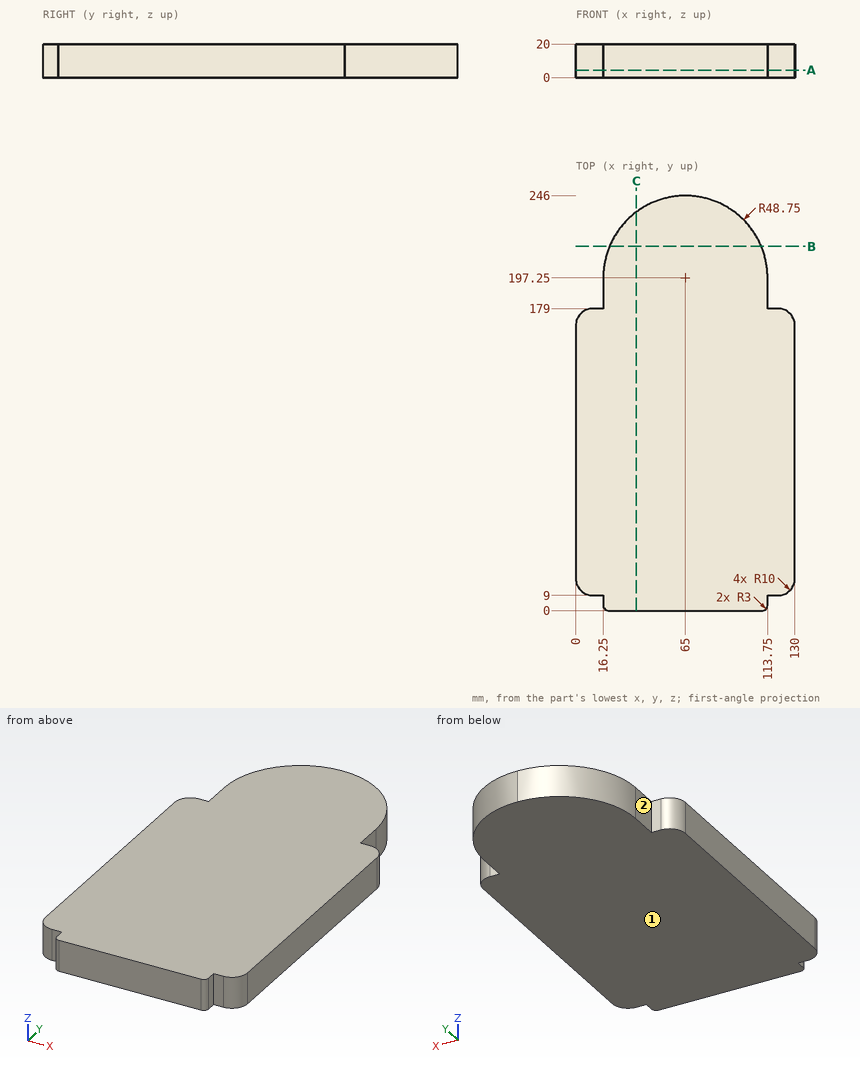
Geometry check sheet. Reference: drawing and pictorial views, mm from the part's lowest x, y, z. A direction names the side the tool comes from. Round coordinates to 2 decimals unless told otherwise and drop trailing zeros. Loops run counter-clockwise (first coordinate to the right, second up) from the corner with the lowest first, then second, coordinate; pieces in that order, holes last. Notation, with made-up numbers: (17.25, 16) -> (22.25, 16) arc R12 ccw to (22.25, 32) -> close; hole circle Ø5 at (-14, 79.25). An arc over 180 degrees is marked (long way). Answer as a JSON object with one key per item and string values. Group by question number.
Item 1: Cross-section at C-C, the plane x = 36. Record the cut outline in (y, z).
Item 2: Depth check by flat-ended pin: pin 1 Ø1.8 at (y, z) = (5, 14) entering from +X; pin 2 Ø4 at (x, z) = (90, 9) entering from +Y; pin 3 Ø1 at (x, z) = (34, 4) entering from +Y. Enter the tip coordinate at first touch or a pass-through.
Item 3: Cross-section at B-B, the plane y = 216. Record the cut outline in (x, z).
Item 4: Thickness scan on line 1 along X through (y, z) = (18, 15.5); line 2 along Y through (x, z) = (117, 4.5); line 3 along Y through (x, z) = (46, 9.5) (3 decimals). Record the ranges inside material, lowest first.
Item 5: Set-up check for the marked faces 1 and 2: record each of +Z, -Z, +X, -X, +Y, -Y from which the full face is reachable in a straight line by a thin tool's end or side.
Item 6: Cross-section at A-A, the plane z = 4.5. Record the cut outline in (x, y), plus the area to 3 significant figures.
Determined:
{
 "1": {"outline": "(0, 0) -> (236.44, 0) -> (236.44, 20) -> (0, 20) -> close"},
 "2": {"pin 1": "stops at x = 113.75", "pin 2": "stops at y = 240.23", "pin 3": "stops at y = 235.28"},
 "3": {"outline": "(20, 0) -> (110, 0) -> (110, 20) -> (20, 20) -> close"},
 "4": {"line 1": "x = 0.05 to 129.95", "line 2": "y = 9 to 179", "line 3": "y = 0 to 242.145"},
 "5": {"face 1": "-Z, +X, -X, +Y, -Y", "face 2": "+Z, -Z, -X, +Y"},
 "6": {"outline": "(0, 19) arc R10 ccw to (10, 9) -> (16.25, 9) -> (16.25, 3) arc R3 ccw to (19.25, 0) -> (110.75, 0) arc R3 ccw to (113.75, 3) -> (113.75, 9) -> (120, 9) arc R10 ccw to (130, 19) -> (130, 169) arc R10 ccw to (120, 179) -> (113.75, 179) -> (113.75, 197.25) arc R48.75 ccw to (65, 246) arc R48.75 ccw to (16.25, 197.25) -> (16.25, 179) -> (10, 179) arc R10 ccw to (0, 169) -> close", "area": "28,400 mm²"}
}
